Verification items for the finished model (mm, model axes). A direction names the side the tool comes from. Coordinates: 2 decimals unless noted, no trailing zeros. Loops run counter-clockwise (first coordinate to the right, second up) from the corner with the lowest first, then second, coordinate; pieces in that order, holes last. Notation, with made-up numbers: (70.25, -24.5) -> (95.25, -24.5) arc R29 ccw to (95.25, 10.5) -> close; hole circle Ø7 at (81.5, 54). An arc over 180 degrees is marked (long way). Answer as a JSON object with one key per item and string values. Group by question number.
Q1. Cross-section at D-D on x = 27.5. Record the boundary of the cut face in (y, z), and give its area (3 significant figures).
Q2. Scan lines: L1, parallel to X at y = 9, z = 23; L2, parallel to X at y = 14, z = 6; L3, parallel to Y at x = 7, z = 4. Record each from-to range of solid material in increasing order.
Q3. Cross-section at B-B on y = 11. Record the boundary of the cut face in (x, z).
Q4. Release check for a two-part mould opening along Z. For faces 1 (the flat face through (-7, 31, 5)), 2 (the cylindrical face through (-4.164, 25.93, 41.675)), 3 (the flat face through (13, 13, 47)) record: released by +Z, released by -Z, zero draft, split by the parting line, or undercut.
Q5. Cross-section at C-C on z = 5. Record the boundary of the cut face in (x, y), and give its area (3 significant figures).
Q6. Cross-section at A-A on z = 25.5. Record the boundary of the cut face in (x, y).
Q7. Set-up check for faces 4 (the cylindrical face through (-7.42, 26.45, 30.43)), 5 (the cylindrical face through (-4.164, 25.93, 16.675)), 6 (the flat face through (-7, 31, 42)): record each of +Z, -Z, +X, -X, +Y, -Y from which the full face is reachable in a straight line by a thin tool's end or side.
Q8. Gauge pin test, flat ends, axial feed: pin 1 Ø5 at (y, z) = (26, 42) entering from +X; pin 2 Ø1 at (y, z) = (25.5, 31.5) entering from -X; pin 3 Ø14 at (x, y) = (5.271, 9.5) entering from -Z; pin 4 Ø4 at (y, z) = (23.5, 16.5) entering from -X. Record the tip position at first contact, or that the pin passes through.
```python
from build123d import *

# Parameters (mm, degrees)
ESQUISSE1_R             = 7.9
BOSS_EXTRU_1_DEPTH      = 47
CONG_1_R                = 5
CONG_2_R                = 5
CONG_4_R                = 3
ESQUISSE2_R             = 2.5
BOSS_EXTRU_2_DEPTH      = 10
ESQUISSE3_R             = 1.5
ENL_V_MAT_EXTRU_1_DEPTH = 6


with BuildPart() as part:
    # Esquisse1 → Boss.-Extru.1 (new body)
    with BuildSketch(Plane.XY):
        with BuildLine():
            ThreePointArc((5.270999392, 0), (14.770999392, 9.5), (5.270999392, 19))
            Line((5.270999392, 19), (49.270999392, 19))
            ThreePointArc((49.270999392, 19), (39.770999392, 9.5), (49.270999392, 0))
            Line((49.270999392, 0), (60.184195152, 0))
            Line((60.184195152, 0), (60.184195152, 21))
            Line((60.184195152, 21), (-11.642273667, 21))
            Line((-11.642273667, 21), (-11.642273667, 0))
            Line((-11.642273667, 0), (5.270999392, 0))
        make_face()
        with Locations((5.270999392, 9.5)):
            Circle(ESQUISSE1_R, mode=Mode.SUBTRACT)
        with Locations((49.270999392, 9.5)):
            Circle(ESQUISSE1_R, mode=Mode.SUBTRACT)
    extrude(amount=BOSS_EXTRU_1_DEPTH)

    # Congé1
    cong_1_edges = [part.edges().sort_by_distance(p)[0] for p in [
        (-11.642273667, 0, 23.5),
    ]]
    fillet(cong_1_edges, radius=CONG_1_R)

    # Congé2
    cong_2_edges = [part.edges().sort_by_distance(p)[0] for p in [
        (60.184195152, 0, 23.5),
    ]]
    fillet(cong_2_edges, radius=CONG_2_R)

    # Congé4
    cong_4_edges = [part.edges().sort_by_distance(p)[0] for p in [
        (60.184195152, 21, 23.5),
    ]]
    fillet(cong_4_edges, radius=CONG_4_R)

    # Esquisse2 → Boss.-Extru.2 (add)
    with BuildSketch(Plane(origin=(0, 21, 0), x_dir=(1, 0, 0), z_dir=(0, 1, 0))):
        with Locations(Location((-6.642273667, -42, 0), (0, 0, 270))):
            Circle(ESQUISSE2_R)
        with Locations(Location((-6.642273667, -29, 0), (0, 0, 270))):
            Circle(ESQUISSE2_R)
        with Locations(Location((-6.642273667, -17, 0), (0, 0, 270))):
            Circle(ESQUISSE2_R)
        with Locations(Location((-6.642273667, -5, 0), (0, 0, 270))):
            Circle(ESQUISSE2_R)
    extrude(amount=BOSS_EXTRU_2_DEPTH)

    # Esquisse3 → Enlèv. mat.-Extru.1 (cut)
    with BuildSketch(Plane.ZY.offset(11.642273667)):
        with Locations((5, 26)):
            Circle(ESQUISSE3_R)
        with Locations((17, 26)):
            Circle(ESQUISSE3_R)
        with Locations((29, 26)):
            Circle(ESQUISSE3_R)
        with Locations((42, 26)):
            Circle(ESQUISSE3_R)
    extrude(amount=-ENL_V_MAT_EXTRU_1_DEPTH, mode=Mode.SUBTRACT)


solid = part.part
```
Computed values:
{
 "1": {"outline": "(19, 0) -> (21, 0) -> (21, 47) -> (19, 47) -> close", "area": "94.0 mm²"},
 "2": {"L1": "x = -11.64 to -2.61, 13.16 to 14.76, 39.78 to 41.39, 57.16 to 60.18", "L2": "x = -11.64 to -1.22, 11.76 to 13.64, 40.9 to 42.78, 55.76 to 60.18", "L3": "y = 0.16 to 1.79, 17.21 to 18.84, 19 to 21"},
 "3": {"outline": "(-11.64, 0) -> (-2.49, 0) -> (-2.49, 47) -> (-11.64, 47) -> close; (13.03, 0) -> (14.65, 0) -> (14.65, 47) -> (13.03, 47) -> close; (39.89, 0) -> (41.51, 0) -> (41.51, 47) -> (39.89, 47) -> close; (57.03, 0) -> (60.18, 0) -> (60.18, 47) -> (57.03, 47) -> close"},
 "4": {"face 1": "zero draft", "face 2": "undercut", "face 3": "released by +Z"},
 "5": {"outline": "(-11.64, 5) arc R5 ccw to (-6.64, 0) -> (5.27, 0) arc R9.5 ccw to (5.27, 19) -> (49.27, 19) arc R9.5 ccw to (49.27, 0) -> (55.18, 0) arc R5 ccw to (60.18, 5) -> (60.18, 18) arc R3 ccw to (57.18, 21) -> (-4.14, 21) -> (-4.14, 31) -> (-9.14, 31) -> (-9.14, 27.5) -> (-5.64, 27.5) -> (-5.64, 24.5) -> (-9.14, 24.5) -> (-9.14, 21) -> (-11.64, 21) -> close; hole circle Ø15.8 at (5.27, 9.5); hole circle Ø15.8 at (49.27, 9.5)", "area": "591 mm²"},
 "6": {"outline": "(-11.64, 5) arc R5 ccw to (-6.64, 0) -> (5.27, 0) arc R9.5 ccw to (5.27, 19) -> (49.27, 19) arc R9.5 ccw to (49.27, 0) -> (55.18, 0) arc R5 ccw to (60.18, 5) -> (60.18, 18) arc R3 ccw to (57.18, 21) -> (-11.64, 21) -> close; hole circle Ø15.8 at (5.27, 9.5); hole circle Ø15.8 at (49.27, 9.5)"},
 "7": {"face 4": "-X", "face 5": "+Y", "face 6": "+Z, -Z, +X, -X, +Y"},
 "8": {"pin 1": "stops at x = -4.14", "pin 2": "stops at x = -8.14", "pin 3": "passes through", "pin 4": "stops at x = -9.14"}
}
